Build history of the part. All positions in model axes, mm. A direction names the side the tool comes from. Round coordinates to 2 decimals unless told otherwise and drop trailing zeros. Order: outer loops, then holes, each group sorted by start corner. A loop starts at its lowest first (then second) coordinate and runs counter-clockwise, first axis right, second up. Notation, with made-up numbers: (-9.75, -32) -> (37.25, -32) arc R8 cw to (37.25, -28) -> close; hole circle Ø6 at (0, -32.75). An arc over 180 degrees is marked (long way). Use a Markdown table: item, result. Add a question column.
Item 1: Slice it at D-D, the plane y = 69.5. Give the cut face in (x, z).
Item 2: 3-axis set-ups, long thin cutter, end or side, ignore diameter. For faces 1 (the face through (-121, 80.158, -60)), 2 (the face through (-84.336, 71.677, -67.686)): which of +Z, -Z, +X, -X, +Y, -Y reach the whole face in a straight line?
Item 3: Slice it at C-C, the plane x = -112. Give the cut face in (y, z), plus the area to 3 significant figures.
Item 4: Two-plate mould, pull along X, no slides. Class faces 3 (the face through (-87.354, 72.894, -67.686)), 4 (the face through (-121, 83.333, -61)), 5 (the face through (-115.188, 79.464, -61.226)), 6 (the face through (-117.22, 81.4, -53.61)): released by +X, released by -X, zero draft, split by the parting line, or undercut.
Item 5: Slice it at A-A, the plane z = -67.25. Give the cut face in (x, y) (1 decimal), plus the area to 3 significant figures.
Item 6: Pin check, flat tips, straight feed: pin 1 (1.9 mm diameter, centred on x = -87.01, y = 74.44, fed in from +Z); pin 2 (1 mm diameter, centred on x = -95.5, z = -67, fed in from +Y); pin 3 (6 mm diameter, centred on x = -96, y = 69.5, fed in from +Z); pin 4 (6 mm diameter, centred on y = 77.5, z = -62.5, fed in from +X). Stop position of each tip, or through.
Item 7: Slice it at B-B, the plane z = -62.5. Give the cut face in (x, y), plus the area to 3 significant figures.
Item 8: Probe L1, parallel to Z at x = -93, y = 73.5; L2, parallel to Y at x = -106.5, z = -64.75; L3, parallel to Y at x = -98.5, z = -68.25. List the from-to ranges inside material, lowest first.
from build123d import *

# Parameters (mm, degrees)
SKETCH1_R           = 1.5875
BOSS_EXTRUDE1_DEPTH = 3.175
BOSS_EXTRUDE2_DEPTH = 12.7
CHAMFER1_SIZE       = 13.716
FILLET1_R           = 3.175


with BuildPart() as part:
    # Sketch1 → Boss-Extrude1 (new body)
    with BuildSketch(Plane.XY.offset(-69.251165667)):
        with BuildLine():
            Line((-122.696825859, 83.333454018), (-119.521825859, 83.333454018))
            Line((-119.521825859, 83.333454018), (-85.973181885, 77.960895375))
            ThreePointArc((-85.973181885, 77.960895375), (-84.441981363, 77.100793683), (-83.834825859, 75.45285189))
            Line((-83.834825859, 75.45285189), (-83.834825859, 73.192832287))
            ThreePointArc((-83.834825859, 73.192832287), (-84.350263921, 71.658964965), (-85.687384095, 70.747628037))
            Line((-85.687384095, 70.747628037), (-119.521825859, 61.235454018))
            Line((-119.521825859, 61.235454018), (-122.696825859, 61.235454018))
            Line((-122.696825859, 61.235454018), (-122.696825859, 83.333454018))
        make_face()
        with Locations((-87.009825859, 74.443454018)):
            Circle(SKETCH1_R, mode=Mode.SUBTRACT)
    extrude(amount=BOSS_EXTRUDE1_DEPTH)

    # Sketch2 → Boss-Extrude2 (add)
    with BuildSketch(Plane.XY.offset(-66.076165667)):
        Polygon((-103.813644634, 77.642908982), (-103.317906173, 80.738520261), (-119.521825859, 83.333454018), (-122.696825859, 83.333454018), (-122.696825859, 80.158454018), (-119.521825859, 80.158454018), align=None)
    extrude(amount=BOSS_EXTRUDE2_DEPTH)

    # Chamfer1
    # the kernel refuses this chamfer: 13.716 mm, written as the material it takes off along each edge
    with BuildSketch(Plane(origin=(-109.391309905, 42.813488073, -53.376165667), x_dir=(0.02714994258719934, -0.004347855574462481, -0.9996219169112966), z_dir=(0.15812754894268197, 0.987418694508758, 0))) as chamfer1_piece_1_section:
        Polygon((CHAMFER1_SIZE * 0.999621916911, CHAMFER1_SIZE * 0.0274958766106), (-CHAMFER1_SIZE * 0.0274958766106, CHAMFER1_SIZE * 0.999621916911), (0, 0), align=None)
    chamfer1_piece_1 = extrude(amount=73.681462081, mode=Mode.PRIVATE)
    chamfer1_piece_1 = split(chamfer1_piece_1, bisect_by=Plane(origin=(-108.089526316, 79.915158718, -66.076165667), z_dir=(0, 0, 1)), keep=Keep.TOP, mode=Mode.PRIVATE)
    add(chamfer1_piece_1, mode=Mode.SUBTRACT)

    # Fillet1
    fillet1_edges = [part.edges().sort_by_distance(p)[0] for p in [
        (-117.109210218, 81.359592083, -53.376165667),
        (-104.568992798, 79.351372211, -66.076165667),
    ]]
    fillet(fillet1_edges, radius=FILLET1_R)


solid = part.part
Check sheet entries:
| question | item | result |
|---|---|---|
| 1 | outline | (-122.7, -69.25) -> (-90.13, -69.25) -> (-90.13, -66.08) -> (-122.7, -66.08) -> close |
| 2 | face 1 | +Z, -X, -Y |
| 2 | face 2 | +Z, -Z, +X, -Y |
| 3 | outline | (63.35, -69.25) -> (82.13, -69.25) -> (82.13, -58.3) -> (78.95, -58.8) -> (78.95, -66.08) -> (63.35, -66.08) -> close |
| 3 | area | 83.5 mm2 |
| 4 | face 3 | undercut |
| 4 | face 4 | zero draft |
| 4 | face 5 | released by -X |
| 4 | face 6 | released by +X |
| 5 | outline | (-122.7, 61.2) -> (-119.5, 61.2) -> (-85.7, 70.7) arc R2.5 ccw to (-83.8, 73.2) -> (-83.8, 75.5) arc R2.5 ccw to (-86, 78) -> (-119.5, 83.3) -> (-122.7, 83.3) -> close; hole circle Ø3.2 at (-87, 74.4) |
| 5 | area | 568 mm2 |
| 6 | pin 1 | through |
| 6 | pin 2 | y = 79.57 |
| 6 | pin 3 | z = -66.08 |
| 6 | pin 4 | x = -105.35 |
| 7 | outline | (-122.7, 80.16) -> (-119.52, 80.16) -> (-108.35, 78.37) -> (-107.85, 81.46) -> (-119.52, 83.33) -> (-122.7, 83.33) -> close |
| 7 | area | 46.3 mm2 |
| 8 | L1 | -69.25 to -66.08 |
| 8 | L2 | 78.07 to 81.25 |
| 8 | L3 | 67.15 to 79.97 |
